Verification items for the finished model (mm, model axes). Face numbers are marked on the shaded views. Coordinates: 2 decimals unless noted, no trailing zeros. Order: outer loops, then holes, each group sorted by start corner. A loop starts at its lowest first (then second) coordinate and runs counter-clockwise, first axis right, second up. Notation, with made-up numbers: (-13.5, 52.25) - (36.5, 52.25) arc R18 ccw to (36.5, 59.25) - close; hole circle Ø1 at (61.5, 71). An arc over 180 degrees is marked (long way). One line per question, with ' | ' between items. Start each with the question number.
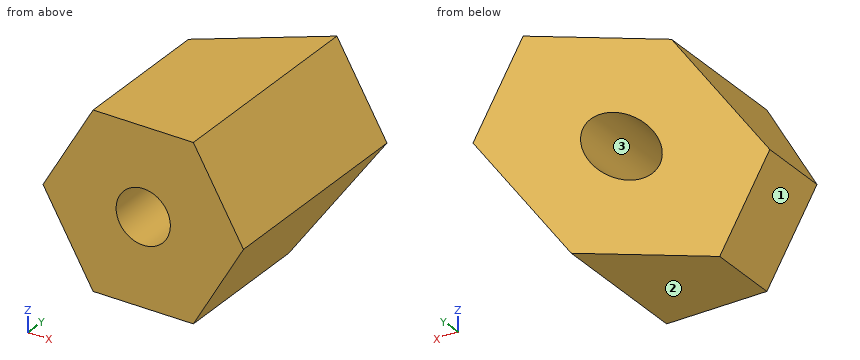
from build123d import *

# Parameters (mm, degrees)
SKETCH1_R           = 12.5
BOSS_EXTRUDE1_DEPTH = 100
DRAFT8_ANGLE        = -40


with BuildPart() as part:
    # Sketch1 → Boss-Extrude1 (new body)
    with BuildSketch(Plane(origin=(0, 0, 0), x_dir=(1, 0, 0), z_dir=(0, 1, 0))):
        Polygon((46.188021535, 0), (23.094010768, 40), (-23.094010768, 40), (-46.188021535, 0), (-23.094010768, -40), (23.094010768, -40), align=None)
        with Locations(Location((0, 0, 0), (0, 0, 270))):
            Circle(SKETCH1_R, mode=Mode.SUBTRACT)
    extrude(amount=BOSS_EXTRUDE1_DEPTH)

    # Draft8
    draft8_faces = [part.faces().sort_by_distance(p)[0] for p in [
        (33.582715627, 100, -19.388989907),
    ]]
    draft(draft8_faces, Plane(origin=(23.094010768, 100, 40), x_dir=(-0.49999999999999944, 0, 0.8660254037844389), z_dir=(0.866025403784439, 0, 0.49999999999999956)), DRAFT8_ANGLE)


solid = part.part
Item 1: Mould release check, pull along X, two halves, no side actions. Record for the marked faces 1, 2 and 3: +X half, -X half, draft (parallel to the pull), parting line (faces both ways), or undercut.
Item 2: Thickness scan on probe 1 along Z at (x, y) = (0, 46); probe 2 along X at (y, z) = (21, 0); probe 3 along Z at (x, y) = (1.5, 57). Record the ranges inside material, lowest first. Write a range as from..to.
Item 3: Section check A-A (y = 29). Record the cut outline in (x, z).
Item 4: Section check D-D (x = -26.5). Record the cut outline in (y, z).
Item 5: Section check B-B (x = 0). Record the cut outline in (y, z).
Item 6: Section check C-C (z = 30.5). Record the cut outline in (x, y), then the cut area to 3 significant figures.
Item 7: Gauge pin test, flat ends, axial feed: pin 1 (1 mm diameter, centred on y = 49, z = 1, fed in from -X); pin 2 (22.5 mm diameter, centred on x = 0, z = 0, fed in from -Y); pin 3 (10 mm diameter, centred on y = 15, z = 17.5, fed in from -X); pin 4 (10 mm diameter, centred on x = 14, z = 24, fed in from +Y). Record the tip position at first contact, or that the pin passes through.
Completed:
1) face 1: -X half | face 2: draft | face 3: undercut
2) probe 1: z = -40..-12.5, 12.5..40 | probe 2: x = -46.19..-12.5, 12.5..46.19 | probe 3: z = -25.09..-12.41, 12.41..40
3) outline: (-46.19, 0) - (-23.09, -40) - (23.09, -40) - (46.19, 0) - (23.09, 40) - (-23.09, 40) - close; hole circle Ø25 at (0, 0)
4) outline: (0, -34.1) - (32.87, -34.1) - (61.49, 34.1) - (0, 34.1) - close
5) outline: (0, -40) - (49.65, -40) - (61.19, -12.5) - (0, -12.5) - close; (0, 12.5) - (71.68, 12.5) - (83.22, 40) - (0, 40) - close
6) outline: (-28.58, 0) - (28.58, 0) - (28.58, 100) - (-28.58, 58.46) - close | area: 4,530 mm^2
7) pin 1: stops at x = -25.32 | pin 2: passes through | pin 3: stops at x = -38.97 | pin 4: stops at y = 90.87
